Source: CAD feature listing. Evaluate the final solid. Frame: model axes, mm. A direction names the side the tool comes from. Coordinates: 2 decimals unless noted, no trailing zeros. Order: outer loops, then holes, each group sorted by start corner. A loop starts at its lowest first (then second) coordinate and runs counter-clockwise, first axis right, second up.
```python
from build123d import *

# Parameters (mm, degrees)
F0_W     = 15.748
F0_H     = 7.7216
F1_DEPTH = 9.5504
F2_R     = 2.4511
F3_DEPTH = 1.905
F4_R     = 2.4511
F5_DEPTH = 1.905
F6_W     = 12.8016
F6_H     = 4.7498
F7_DEPTH = 7.62
F8_R     = 1.4859
F9_DEPTH = 7.62


with BuildPart() as f1:
    # F0 (on Top) → F1 (new body)
    with BuildSketch(Plane.XY):
        Rectangle(F0_W, F0_H)
    extrude(amount=F1_DEPTH)

    # F2 (on face) → F3 (join)
    with BuildSketch(Plane.XY.offset(9.5504)):
        with Locations((-3.6957, 0.0127)):
            Circle(F2_R)
    extrude(amount=F3_DEPTH)

    # F4 (on face) → F5 (join)
    with BuildSketch(Plane.XY.offset(9.5504)):
        with Locations((3.6957, 0.0127)):
            Circle(F4_R)
    extrude(amount=F5_DEPTH)

    # F6 (on face) → F7 (cut)
    with BuildSketch(Plane(origin=(0, 0, 0), x_dir=(1, 0, 0), z_dir=(0, 0, -1))):
        Rectangle(F6_W, F6_H)
    extrude(amount=-F7_DEPTH, mode=Mode.SUBTRACT)

    # F8 (on face) → F9 (join)
    with BuildSketch(Plane(origin=(0, 0, 7.62), x_dir=(1, 0, 0), z_dir=(0, 0, -1))):
        Circle(F8_R)
    extrude(amount=F9_DEPTH)


solid = f1.part
```
Q1. Pull-direction query (Y, two-part tool) for faces 1 (the cylindrical face through (1.417, -0.446, 3.863)), 2 (the flat face through (0, 3.861, 5)), 3 (the flat face through (0, 0, 0)); classes: pulls with the +Y half, pulls with the -Y half, needs draft (parallel to the pull), parting line crosses it, or undercut.
Solutions:
face 1: undercut
face 2: pulls with the +Y half
face 3: needs draft
Q2. Material intervals for line 1 along X through (y, z) = (-0.75, 0.75); line 2 along X through (y, z) = (1.25, 5.5); line 3 along Y through (x, z) = (6.25, 6.25), sorted ascending.
Solutions:
line 1: x = -7.87 to -6.4, -1.28 to 1.28, 6.4 to 7.87
line 2: x = -7.87 to -6.4, -0.8 to 0.8, 6.4 to 7.87
line 3: y = -3.86 to -2.37, 2.37 to 3.86
Q3. Set-up query: faces 4 (the flat face through (0, 0, 9.55)), 5 (the flat face through (-6.401, 0, 4)), 6 (the flat face through (-4, 0, 11.455)). Return all of +Z, -Z, +X, -X, +Y, -Y with unobstructed straight access to the full face (end or side cutting, diameter ignored); none if empty.
Solutions:
face 4: +Z
face 5: -Z
face 6: +Z, +X, -X, +Y, -Y
Q4. Section query D-D on x = -3.75. Output: boundary loops of the cut face in (y, z).
Solutions:
outline: (-3.86, 0) - (-2.37, 0) - (-2.37, 7.62) - (2.37, 7.62) - (2.37, 0) - (3.86, 0) - (3.86, 9.55) - (2.46, 9.55) - (2.46, 11.46) - (-2.44, 11.46) - (-2.44, 9.55) - (-3.86, 9.55) - close
Q5. Section query C-C on y = -2. Output: boundary loops of the cut face in (x, z).
Solutions:
outline: (-7.87, 0) - (-6.4, 0) - (-6.4, 7.62) - (6.4, 7.62) - (6.4, 0) - (7.87, 0) - (7.87, 9.55) - (5.09, 9.55) - (5.09, 11.46) - (2.3, 11.46) - (2.3, 9.55) - (-2.3, 9.55) - (-2.3, 11.46) - (-5.09, 11.46) - (-5.09, 9.55) - (-7.87, 9.55) - close
Q6. Section query A-A on z = 5.25. Output: boundary loops of the cut face in (x, y), plus the area to 3 significant figures.
Solutions:
outline: (-7.87, -3.86) - (7.87, -3.86) - (7.87, 3.86) - (-7.87, 3.86) - close; circle Ø2.97 at (0, 0); hole (-6.4, -2.37) - (6.4, -2.37) - (6.4, 2.37) - (-6.4, 2.37) - close
area: 67.7 mm2
Q7. Section query B-B on x = 0. Output: boundary loops of the cut face in (y, z), plus the area to 3 significant figures.
Solutions:
outline: (-3.86, 0) - (-2.37, 0) - (-2.37, 7.62) - (-1.49, 7.62) - (-1.49, 0) - (1.49, 0) - (1.49, 7.62) - (2.37, 7.62) - (2.37, 0) - (3.86, 0) - (3.86, 9.55) - (-3.86, 9.55) - close
area: 60.2 mm2
